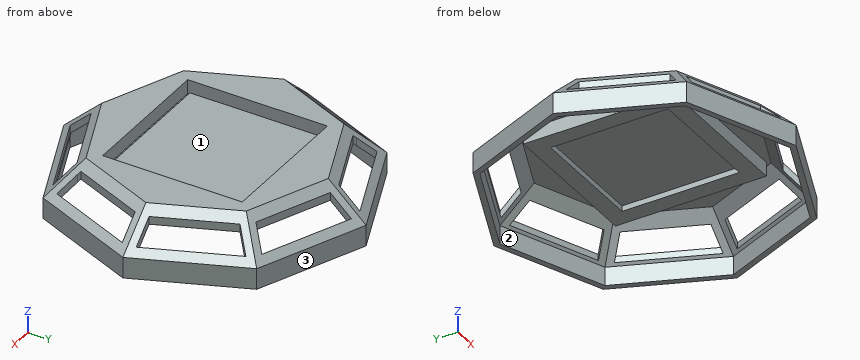
```python
from build123d import *

# Parameters (mm, degrees)
F1_DEPTH = 40
F2_SIZE  = 25
F3_W     = 100
F3_H     = 100
F4_DEPTH = 10
F5_W     = 92
F5_H     = 92
F6_DEPTH = 4
F7_T     = -4
F9_DEPTH = 25


with BuildPart() as f1:
    # F0 (on Top) → F1 (new body)
    with BuildSketch(Plane.XY):
        Polygon((108.2392200292, 0), (76.536686473, 76.536686473), (0, 108.2392200292), (-76.536686473, 76.536686473), (-108.2392200292, 0), (-76.536686473, -76.536686473), (0, -108.2392200292), (76.536686473, -76.536686473), align=None)
    extrude(amount=F1_DEPTH)

    # F2
    f2_edges = [f1.edges().sort_by_distance(p)[0] for p in [
        (38.268343, 92.387953, 40),
        (-38.268343, 92.387953, 40),
        (-92.387953, 38.268343, 40),
        (-92.387953, -38.268343, 40),
        (-38.268343, -92.387953, 40),
        (38.268343, -92.387953, 40),
        (92.387953, -38.268343, 40),
        (92.387953, 38.268343, 40),
    ]]
    chamfer(f2_edges, length=F2_SIZE)

    # F3 (on face) → F4 (cut)
    with BuildSketch(Plane.XY.offset(40)):
        Rectangle(F3_W, F3_H)
    extrude(amount=-F4_DEPTH, mode=Mode.SUBTRACT)

    # F5 (on face) → F6 (join)
    with BuildSketch(Plane.XY.offset(30)):
        Rectangle(F5_W, F5_H)
    extrude(amount=F6_DEPTH)

    # F7
    f7_openings = [f1.faces().sort_by_distance(p)[0] for p in [
        (0, 0, 0),
    ]]
    offset(amount=F7_T, openings=f7_openings, kind=Kind.INTERSECTION)

    # F8 (on face) → F9 (cut)
    with BuildSketch(Plane.XY.offset(40)):
        Polygon((-67.7146268432, -74.7856946551), (-5, -100.7629436527), (-5, -87.6805206605), (-5, -85.6094528486), (-56.999490737, -64.0705585489), (-58.4639568311, -65.5350246429), align=None)
        Polygon((5.000001811, -100.7629429025), (67.7146250322, -74.7856954052), (58.4639555505, -65.5350259235), (56.999488926, -64.070559299), (5.000001811, -85.6094520985), (5.000001811, -87.6805206605), align=None)
        Polygon((65.5350259235, 58.4639555505), (64.070559299, 56.999488926), (85.6094520985, 5.000001811), (87.6805206605, 5.000001811), (100.7629429025, 5.000001811), (74.7856954052, 67.7146250322), align=None)
        Polygon((56.999490737, 64.0705585489), (58.4639568311, 65.5350246429), (67.7146268432, 74.7856946551), (5.000001811, 100.7629429025), (5.000001811, 87.6805206605), (5.000001811, 85.6094520985), align=None)
        Polygon((-67.7146268432, 74.7856946551), (-58.4639568311, 65.5350246429), (-56.999490737, 64.0705585489), (-5, 85.6094528486), (-5, 87.6805206605), (-5, 100.7629436527), align=None)
        Polygon((74.7856946551, -67.7146268432), (100.7629436527, -5), (87.6805206605, -5), (85.6094528486, -5), (64.0705585489, -56.999490737), (65.5350246429, -58.4639568311), align=None)
        Polygon((-74.7856954052, 67.7146250322), (-100.7629429025, 5.000001811), (-87.6805206605, 5.000001811), (-85.6094520985, 5.000001811), (-64.070559299, 56.999488926), (-65.5350259235, 58.4639555505), align=None)
        Polygon((-100.7629436527, -5), (-74.7856954052, -67.7146250322), (-65.5350259235, -58.4639555505), (-64.070559299, -56.999488926), (-85.6094528486, -5), (-87.6805206605, -5), align=None)
    extrude(amount=-F9_DEPTH, mode=Mode.SUBTRACT)


solid = f1.part
```
Could you check a few things on this model? Use its own coordinates, in mm. Face numbers are marked on the shaded views. A direction names the side the tool comes from. Round coordinates to 2 decimals unless told otherwise and drop trailing zeros. Loops run counter-clockwise (first coordinate to the right, second up) from the corner with the lowest first, then second, coordinate; pieces in that order, holes last.
Q1. I want a section at D-D (y = 2.5). Write out the boundary of the cut face in (x, z), and give its area (3 significant figures).
Q2. I want a section at B-B (z = 10.5). Write out the boundary of the cut face in (x, y).
Q3. I want a section at C-C (x = 12.5). Give the number of separate pieces and of enclosed holes in the cut face, and give its area (3 significant figures).
Q4. On a 3-axis mill with a long thin cutter (end or side, diameter ignored), from which of +Z, -Z, +X, -X, +Y, -Y can I reach the whole of each face in a straight line? I mean the marked faces 1, 2 and 3. Say none if no direction works.
Q5. I want a section at A-A (y = -92). Write out the boundary of the cut face in (x, z), and give its area (3 significant figures).
Q6. For P1, Ø12, axis at x = 96, z = 27.5, coming from the +Y side; P2, Ø5, axis at x = 20.5, y = -58.5, coming from the -Z side; P3, Ø3, axis at y = -14.5, z = 33, coming from the -X side, each with a flat end and sliding along its axis, tell me the tip position at first contact or that it passes through.
Q7. Please list where these lines run through material, in increasing order: L1, parallel to X at y = 42, z = 33.5; L2, parallel to Z at x = 59.5, y = -45.5; L3, parallel to Z at x = -29.5, y = 23.5.
Answer below:
1. outline: (-107.2, 0) - (-102.87, 0) - (-102.87, 13.34) - (-78.35, 36) - (-54, 36) - (-54, 26) - (-42, 26) - (-42, 30) - (42, 30) - (42, 26) - (54, 26) - (54, 36) - (78.35, 36) - (102.87, 13.34) - (102.87, 0) - (107.2, 0) - (107.2, 15) - (80.14, 40) - (50, 40) - (50, 30) - (46, 30) - (46, 34) - (-46, 34) - (-46, 30) - (-50, 30) - (-50, 40) - (-80.14, 40) - (-107.2, 15) - close
1. area: 1,160 mm2
2. outline: (-108.24, 0) - (-76.54, -76.54) - (0, -108.24) - (76.54, -76.54) - (108.24, 0) - (76.54, 76.54) - (0, 108.24) - (-76.54, 76.54) - close; hole (-103.91, 0) - (-73.48, -73.48) - (0, -103.91) - (73.48, -73.48) - (103.91, 0) - (73.48, 73.48) - (0, 103.91) - (-73.48, 73.48) - close
3. separate pieces: 3
3. enclosed holes: 0
3. area: 956 mm2
4. face 1: +Z
4. face 2: -Z
4. face 3: +Z, -Z, +X, +Y
5. outline: (-39.2, 0) - (-28.75, 0) - (-28.75, 13.34) - (-24.42, 15) - (-26.16, 15) - (-26.16, 19.99) - (-39.2, 15) - close; (-5, 22.43) - (0, 24.35) - (5, 22.43) - (5, 28.09) - (0, 30) - (-5, 28.09) - close; (24.42, 15) - (28.75, 13.34) - (28.75, 0) - (39.2, 0) - (39.2, 15) - (26.16, 19.99) - (26.16, 15) - close
5. area: 442 mm2
6. P1: stops at y = 5
6. P2: stops at z = 36
6. P3: stops at x = -82.3
7. L1: x = -70.28 to -64.7, -54 to -50, -46 to 46, 50 to 54, 64.7 to 70.28
7. L2: z = 36 to 40
7. L3: z = 30 to 34
